from build123d import *

# Parameters (mm, degrees)
F0_W      = 50
F0_H      = 10
F1_DEPTH  = 5
F0_W_2    = 5
F0_H_2    = 80
F2_DEPTH  = 55
F3_W      = 15
F3_H      = 5
F4_DEPTH  = 125
F6_W      = 5
F6_H      = 15
F5_W      = 5
F5_H      = 15
F7_DEPTH  = 50
F8_R      = 4.99999
F10_DEPTH = 80.001


# Not quite as in the source:
# - a fillet or chamfer is up to 0.001 mm smaller than in the source, because OpenCascade refuses the exact size


with BuildPart() as f1:
    # F0 (on Top) → F1 (new body)
    with BuildSketch(Plane.XY):
        Polygon((59.8684251308, 39.4171364857), (14.8684251308, 39.4171364857), (14.8684251308, -40.5828635143), (59.8684251308, -40.5828635143), (59.8684251308, -30.5828635143), (59.8684251308, -20.5828635143), (59.8684251308, -10.5828635143), (59.8684251308, -5.5828635143), (59.8684251308, 4.4171364857), (59.8684251308, 9.4171364857), (59.8684251308, 19.4171364857), (59.8684251308, 29.4171364857), align=None)
        with Locations((84.8684251308, -0.5828635143)):
            Rectangle(F0_W, F0_H)
        with Locations((84.8684251308, -35.5828635143)):
            Rectangle(F0_W, F0_H)
        with Locations((84.8684251308, 14.4171364857)):
            Rectangle(F0_W, F0_H)
        with Locations((84.8684251308, 34.4171364857)):
            Rectangle(F0_W, F0_H)
        with Locations((84.8684251308, -15.5828635143)):
            Rectangle(F0_W, F0_H)
    extrude(amount=F1_DEPTH)

    # F0 (on Top) → F2 (join)
    with BuildSketch(Plane.XY):
        with Locations((12.3684251308, -0.5828635143)):
            Rectangle(F0_W_2, F0_H_2)
    extrude(amount=F2_DEPTH)

    # F3 (on face) → F4 (join)
    with BuildSketch(Plane(origin=(9.8684251308, 0, 0), x_dir=(0, -1, 0), z_dir=(-1, 0, 0))):
        with Locations((-31.9171364857, 52.5)):
            Rectangle(F3_W, F3_H)
        with Locations((33.0828635143, 52.5)):
            Rectangle(F3_W, F3_H)
    extrude(amount=F4_DEPTH)

    # F6 (on face) + F5 (on face) → F7 (join)
    with BuildSketch(Plane(origin=(0, 0, 50), x_dir=(1, 0, 0), z_dir=(0, 0, -1))):
        with Locations((-112.6315748692, 33.0828635143)):
            Rectangle(F6_W, F6_H)
    with BuildSketch(Plane(origin=(0, 0, 50), x_dir=(1, 0, 0), z_dir=(0, 0, -1))):
        with Locations((-112.6315748692, -31.9171364857)):
            Rectangle(F5_W, F5_H)
    extrude(amount=F7_DEPTH)

    # F8 (radius 5 in the source; OpenCascade refuses exactly that, so slightly less here)
    f8_edges = [f1.edges().sort_by_distance(p)[0] for p in [
        (-115.131575, 31.917136, 55),
        (-115.131575, -33.082864, 55),
        (9.868425, -0.582864, 0),
        (14.868425, -0.582864, 55),
    ]]
    fillet(f8_edges, radius=F8_R)

    # F9 (on face) → F10 (cut, through all)
    with BuildSketch(Plane.XZ.offset(40.5828635143)):
        with BuildLine():
            add(Edge.make_bspline(
                [(107.8684251308, 5), (106.7611965953, 3.8240237002), (103.011923181, 1.9991854383), (101.7375563624, 4.0782074875), (100.8684251308, 5)],
                knots=[0, 0, 0, 0, 0.5536142678, 1, 1, 1, 1], degree=3))
            Line((107.8684251308, 5), (100.8684251308, 5))
        make_face()
    extrude(amount=-F10_DEPTH, mode=Mode.SUBTRACT)


solid = f1.part
Geometry check sheet. Reference: the model listing, model coordinates, mm. A direction names the side the tool comes from. Coordinates: 2 decimals unless noted, no trailing zeros. Loops run counter-clockwise (first coordinate to the right, second up) from the corner with the lowest first, then second, coordinate; pieces in that order, holes last. Notation, with made-up numbers: (29.25, -28) - (52.25, -28) arc R18 cw to (52.25, 2) - close; hole circle Ø1 at (6, 60). An arc over 180 degrees is marked (long way). Use one line per item in the form item = value. Start each with the question number.
Item 1: Thickness scan on probe 1 along X at (y, z) = (27.5, 44); probe 2 along Y at (x, z) = (-93, 51); probe 3 along Z at (x, y) = (77.5, -1). Record the ranges inside material, lowest first.
Item 2: Section check C-C, the plane x = 2. Enter the section's corners in (y, z).
Item 3: Mould release check, pull along X, two halves, no side actions. Record for faces 4 (the face through (85, -30.583, 2)), 5 (the face through (-49, -33, 50)), 6 (the face through (109.868, 34, 2)): +X half, -X half, draft (parallel to the pull), parting line (faces both ways), or undercut.
Item 4: Section check A-A, the plane z = 27. Enter the section's corners in (x, y), and give its area (3 significant figures).
Item 5: Tool access check on faces 1 (the face through (-71, 24.417, 52)), 2 (the face through (14.868, -1, 27)), 3 (the face through (85, 9.417, 2)). Record the directions out of +Z, -Z, +X, -X, +Y, -Y that give a thin tool (end or side, any length) a straight path to the whole face; none if there is none.
Item 6: Section check B-B, the plane x = 86. Enter the section's corners in (y, z), and give its area (3 significant figures).
Item 7: Gauge pin test, flat ends, axial feed: pin 1 (10 mm diameter, centred on x = 81, y = -20.5, fed in from +Z); pin 2 (13.5 mm diameter, centred on y = 16, z = 17.5, fed in from +X); pin 3 (16.5 mm diameter, centred on x = -28.5, y = 34.5, fed in from -Z). Record the tip position at first contact, or that the pin passes through.
Computed:
q1.probe_1 = -115.13 to -110.13, 9.87 to 14.87
q1.probe_2 = -40.58 to -25.58, 24.42 to 39.42
q1.probe_3 = 0 to 5
q2.outline = (-40.58, 50) - (-25.58, 50) - (-25.58, 55) - (-40.58, 55) - close; (24.42, 50) - (39.42, 50) - (39.42, 55) - (24.42, 55) - close
q3.face_4 = draft
q3.face_5 = undercut
q3.face_6 = +X half
q4.outline = (-115.13, -40.58) - (-110.13, -40.58) - (-110.13, -25.58) - (-115.13, -25.58) - close; (-115.13, 24.42) - (-110.13, 24.42) - (-110.13, 39.42) - (-115.13, 39.42) - close; (9.87, -40.58) - (14.87, -40.58) - (14.87, 39.42) - (9.87, 39.42) - close
q4.area = 550 mm2
q5.face_1 = +Z, -Z, -X
q5.face_2 = +Z, +X, +Y, -Y
q5.face_3 = +Z, -Z, +X
q6.outline = (-40.58, 0) - (-30.58, 0) - (-30.58, 5) - (-40.58, 5) - close; (-20.58, 0) - (-10.58, 0) - (-10.58, 5) - (-20.58, 5) - close; (-5.58, 0) - (4.42, 0) - (4.42, 5) - (-5.58, 5) - close; (9.42, 0) - (19.42, 0) - (19.42, 5) - (9.42, 5) - close; (29.42, 0) - (39.42, 0) - (39.42, 5) - (29.42, 5) - close
q6.area = 250 mm2
q7.pin_1 = 5
q7.pin_2 = 14.87
q7.pin_3 = 50
